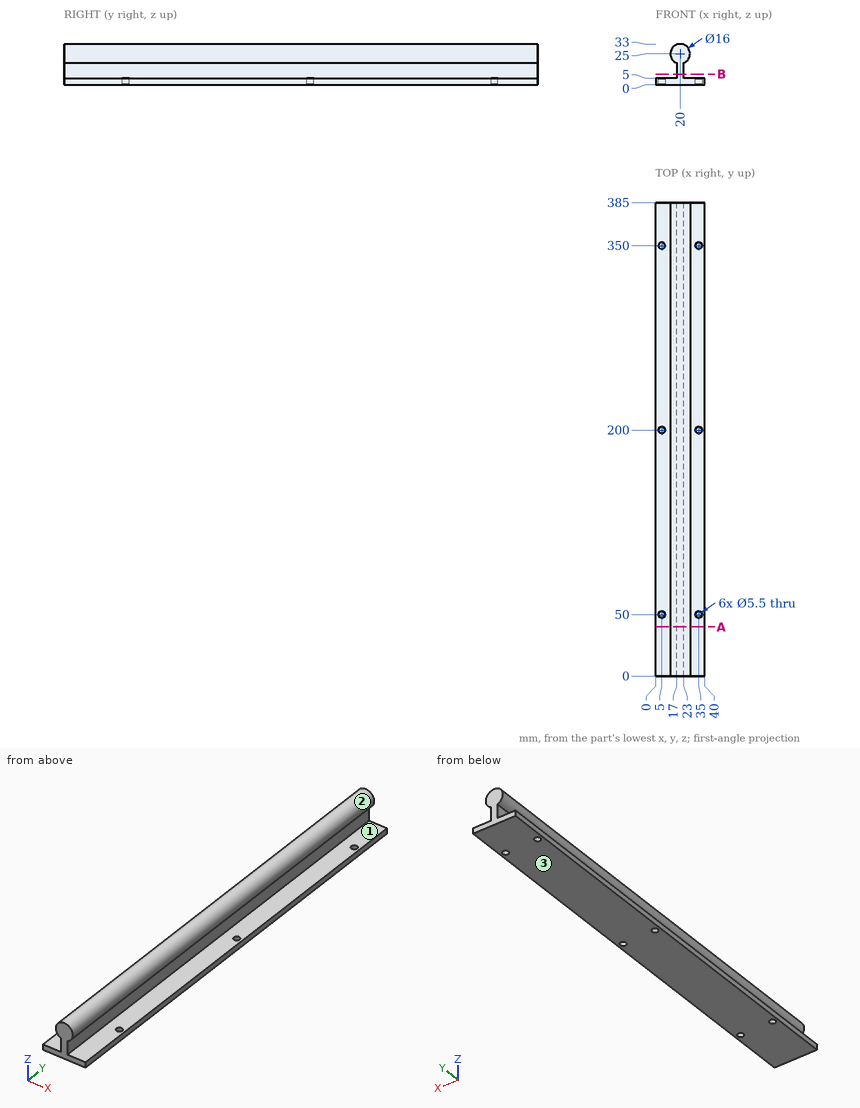
Could you check a few things on this drawing? It's one solid part, dimensions in mm from its lowest x, y, z. Give positions to 0.01 mm unless a question says otherwise; leave off trailing zeros. Order: outer loops, then holes, each group sorted by start corner. A loop starts at its lowest first (then second) coordinate and runs counter-clockwise, first axis right, second up. Notation, with made-up numbers: (55.25, 67) - (91.25, 67) arc R30 ccw to (91.25, 104) - close; hole circle Ø8 at (65.25, 54). An arc over 180 degrees is marked (long way). One line per question, with ' | ' between items. Start each with the question number.
Item 1: Thinking about a two-plate mould opening in Z: for the marked faces 1, 2 and 3, which applies, pulls with the +Z half, pulls with the -Z half, needs draft (parallel to the pull), parting line crosses it, or undercut?
Item 2: I want a section at A-A on y = 40. Write out the boundary of the cut face in (x, z), then the cut area to 3 significant figures.
Item 3: I want a section at B-B on z = 8.5. Write out the boundary of the cut face in (x, y), then the cut area to 3 significant figures.
Item 4: I need wall thicknesses on probe 1 along X at (y, z) = (200, 2); probe 2 along Y at (x, z) = (5, 1); probe 3 along Z at (x, y) = (31.5, 92). Which ranges of each line are inside material? Lowest first, please. Write a range as [from, to].
Item 5: I'm going to push flat-ended pins straight in: pin 1 Ø6.5 at (y, z) = (227.5, 9) entering from +X; pin 2 Ø8.5 at (x, y) = (11, 145.5) entering from +Z; pin 3 Ø7 at (x, y) = (35, 200) entering from -Z; pin 4 Ø18.5 at (x, y) = (32, 102) entering from +Z. Where does each tip first touch, or does it pass through?
Verdict:
1) face 1: undercut | face 2: undercut | face 3: pulls with the -Z half
2) outline: (0, 0) - (40, 0) - (40, 5) - (23, 5) - (23, 17.58) arc R8 ccw (long way) to (17, 17.58) - (17, 5) - (0, 5) - close | area: 474 mm^2
3) outline: (17, 0) - (23, 0) - (23, 385) - (17, 385) - close | area: 2,310 mm^2
4) probe 1: [0, 2.25], [7.75, 32.25], [37.75, 40] | probe 2: [0, 47.25], [52.75, 197.25], [202.75, 347.25], [352.75, 385] | probe 3: [0, 5]
5) pin 1: x = 23 | pin 2: z = 31.44 | pin 3: z = 0 | pin 4: z = 32.51
